Source: CAD feature listing. Evaluate the final solid. Frame: model axes, mm. Face numbers are marked on the shaded views. A direction names the side the tool comes from. Coordinates: 2 decimals unless noted, no trailing zeros. Order: outer loops, then holes, each group sorted by start corner. A loop starts at its lowest first (then second) coordinate and runs counter-clockwise, first axis right, second up.
```python
from build123d import *

# Parameters (mm, degrees)
F0_R      = 6.3
F1_DEPTH  = 10
F1_TAPER  = 2
F0_R_2    = 7.5
F1_FACE_R = 6.3
F2_DEPTH  = 1.5
F3_SIZE   = 0.3
F4_T      = -1.5


# Not quite as in the source:
# - a fillet or chamfer that OpenCascade refuses, or shapes differently, is made with other operations: its cross-section is extruded or revolved along the edge and cut away or added


with BuildPart() as f1:
    # F0 (on Front) → F1 (new body)
    with BuildSketch(Plane.XZ):
        Circle(F0_R)
    extrude(amount=F1_DEPTH, taper=F1_TAPER)

    # F0 (on Front) + F1_face (on face) → F2 (join)
    with BuildSketch(Plane.XZ):
        Circle(F0_R_2)
        Circle(F0_R, mode=Mode.SUBTRACT)
    with BuildSketch(Plane(origin=(0, 0, 0), x_dir=(1, 0, 0), z_dir=(0, 1, 0))):
        Circle(F1_FACE_R)
    extrude(amount=-F2_DEPTH, dir=(0, -1, 0))

    # F3
    f3_edges = [f1.edges().sort_by_distance(p)[0] for p in [
        (-7.5, 1.5, 0),
    ]]
    chamfer(f3_edges, length=F3_SIZE)

    # F4
    f4_openings = [f1.faces().sort_by_distance(p)[0] for p in [
        (0, -10, 0),
    ]]
    offset(amount=F4_T, openings=f4_openings, kind=Kind.INTERSECTION)

    # F5: chamfer of 0.5 on 1 edges, made by hand

    # F5_s1 → F5_t2 (revolve, cut)
    with BuildSketch(Plane.XY):
        Polygon((5.9682420534, -9.5003045865), (5.4507923051, -10), (5.9507923051, -10), align=None)
    revolve(axis=Axis((0, -10, 0), (0, 1, 0)), mode=Mode.SUBTRACT)


solid = f1.part
```
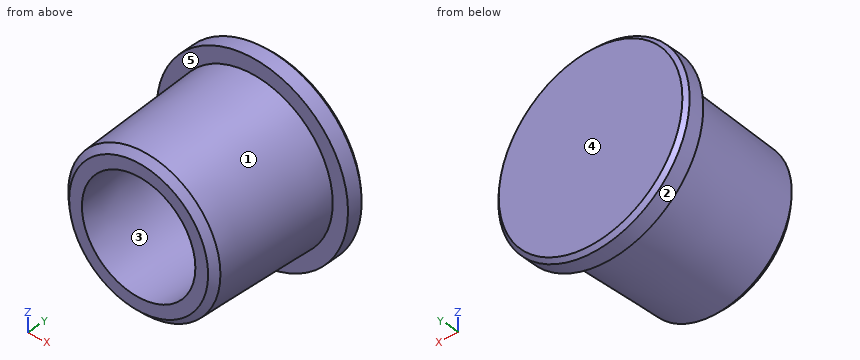
1. Ray query, line 1 (Y direction, x = 3.5, z = 2.25); line 2 (Z direction, x = 3.5, y = -2.75); line 3 (X direction, y = -6.25, z = 3.75). Return the intervals inside material, ascending.
Findings:
line 1: y = 0 to 1.5
line 2: z = -5.12 to -3.14, 3.14 to 5.12
line 3: x = -4.79 to -2.63, 2.63 to 4.79
2. Draft query along Y for the marked faces 3, 4 and 5. Return one class per face: released by +Y, released by -Y, zero draft, split by the parting line, or undercut.
Findings:
face 3: undercut
face 4: released by +Y
face 5: released by -Y
3. Section query C-C on y = -8.75. Return loops of the section in (x, z).
Findings:
outline: circle Ø11.99 at (0, 0); hole circle Ø8.99 at (0, 0)
4. Pin query (flat end, axial travel): P1, Ø5, axis at x = -4, y = 0, coming from the +Z side; P2, Ø2, axis at x = 5.5, y = -2.5, coming from the +Z side; P3, Ø1, axis at x = 0.5, y = -2.5, coming from the -Z side. Return the tip coordinate at first contact, or that it passes through.
Findings:
P1: stops at z = 7.35
P2: stops at z = 4.28
P3: stops at z = -6.22
5. Section query B-B on y = -6. Return loops of the section in (x, z), plus the area to 3 significant figures.
Findings:
outline: circle Ø12.18 at (0, 0); hole circle Ø9.18 at (0, 0)
area: 50.4 mm2
6. Section query A-A on x = 0. Return loops of the section in (y, z), plus the area to 3 significant figures.
Findings:
outline: (-10, -5.45) - (-9.5, -5.97) - (0, -6.3) - (0, -7.5) - (1.2, -7.5) - (1.5, -7.2) - (1.5, 7.2) - (1.2, 7.5) - (0, 7.5) - (0, 6.3) - (-9.5, 5.97) - (-10, 5.45) - (-10, 4.45) - (0, 4.8) - (0, -4.8) - (-10, -4.45) - close
area: 52.2 mm2
7. Access query for the marked faces 1 and 2. Directions: +Z, -Z, +X, -X, +Y, -Y. A direction counts if a zero-diameter tool reaches every point of the face in a straight line with its end or side. Return the directions, or none.
Findings:
face 1: -Y
face 2: +Y, -Y
